Here's how the part is built. I have some questions about the finished solid (model axes, mm). Face numbers are marked on the shaded views. A direction names the side the tool comes from. Give positions to 0.01 mm unless a question says otherwise; leave off trailing zeros. Loops run counter-clockwise (first coordinate to the right, second up) from the corner with the lowest first, then second, coordinate; pieces in that order, holes last. Notation, with made-up numbers: M 43.5,71.5 L 72.5,71.5 A14 ccw 72.5,83.5 Z; hole C 30,-12 d3. An arc over 180 degrees is marked long. Write item = value, one per line. Start each with the question number.
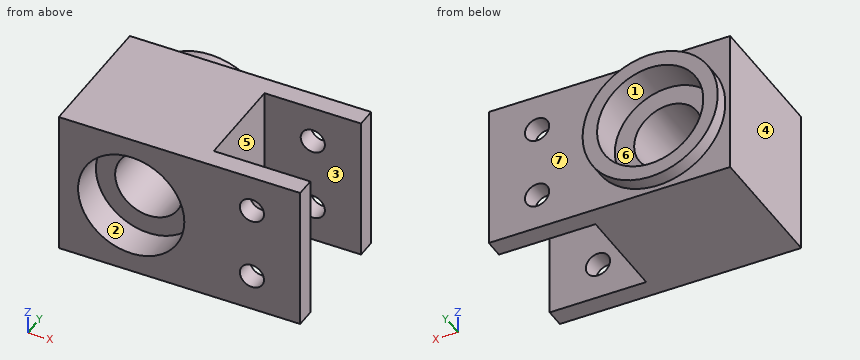
```python
from build123d import *

# Parameters (mm, degrees)
BOSS_EXTRUDE1_DEPTH = 30
SKETCH2_R           = 7
CUT_EXTRUDE1_DEPTH  = 29
SKETCH3_R           = 11
CUT_EXTRUDE2_DEPTH  = 4
SKETCH4_R           = 11
CUT_EXTRUDE3_DEPTH  = 7
SKETCH5_R           = 2.5
CUT_EXTRUDE4_DEPTH  = 29
SKETCH6_R           = 14
SKETCH6_R_2         = 11
BOSS_EXTRUDE2_DEPTH = 3


with BuildPart() as part:
    # Sketch1 → Boss-Extrude1 (new body)
    with BuildSketch(Plane.XY):
        Polygon((10, 10), (10, 14), (-40, 14), (-40, -14), (10, -14), (10, -10), (-10, -10), (-10, 10), align=None)
    extrude(amount=BOSS_EXTRUDE1_DEPTH)

    # Sketch2 → Cut-Extrude1 (cut, through all)
    with BuildSketch(Plane(origin=(0, 14, 0), x_dir=(1, 0, 0), z_dir=(0, 1, 0))):
        with Locations((-25, -15)):
            Circle(SKETCH2_R)
    extrude(amount=-CUT_EXTRUDE1_DEPTH, mode=Mode.SUBTRACT)

    # Sketch3 → Cut-Extrude2 (cut)
    with BuildSketch(Plane(origin=(0, 14, 0), x_dir=(1, 0, 0), z_dir=(0, 1, 0))):
        with Locations((-25, -15)):
            Circle(SKETCH3_R)
    extrude(amount=-CUT_EXTRUDE2_DEPTH, mode=Mode.SUBTRACT)

    # Sketch4 → Cut-Extrude3 (cut)
    with BuildSketch(Plane.XZ.offset(14)):
        with Locations((-25, 15)):
            Circle(SKETCH4_R)
    extrude(amount=-CUT_EXTRUDE3_DEPTH, mode=Mode.SUBTRACT)

    # Sketch5 → Cut-Extrude4 (cut, through all)
    with BuildSketch(Plane(origin=(0, 14, 0), x_dir=(1, 0, 0), z_dir=(0, 1, 0))):
        with Locations((0, -22.5)):
            Circle(SKETCH5_R)
        with Locations((0, -7.5)):
            Circle(SKETCH5_R)
    extrude(amount=-CUT_EXTRUDE4_DEPTH, mode=Mode.SUBTRACT)

    # Sketch6 → Boss-Extrude2 (add)
    with BuildSketch(Plane(origin=(0, 14, 0), x_dir=(1, 0, 0), z_dir=(0, 1, 0))):
        with Locations((-25, -15)):
            Circle(SKETCH6_R)
        with Locations((-25, -15)):
            Circle(SKETCH6_R_2, mode=Mode.SUBTRACT)
    extrude(amount=BOSS_EXTRUDE2_DEPTH)


solid = part.part
```
Q1. If I drill on line 1 along Y through (x, z) = (-1, 18.5); line 2 along Z through (x, y) = (0, 12); line 3 along X through (y, z) = (-11.2, 7.5), over which ranges is the centre line in solid material (lowest first)?
Q2. On a 3-axis mill with a long thin cutter (end or side, diameter ignored), from which of +Z, -Z, +X, -X, +Y, -Y can I reach the whole of each face in a straight line? I mean the marked faces 1, 2 and 3. Say none if no direction works.
Q3. If we section it at D-D, the plane y = 13: List the corners of the cut face in (x, z) for me.
Q4. If we section it at C-C, the plane y = -1.5: List the corners of the cut face in (x, z) for me.
Q5. If we section it at B-B, the plane z = 15: List the corners of the cut face in (x, y) for me, then the cut area to 3 significant figures.
Q6. We'd pull the mould along X, two halves only. Please class the marked faces 4, 5, 6 and 7: pulls with the +X half, pulls with the -X half, needs draft (parallel to the pull), parting line crosses it, or undercut.
Q7. If we section it at A-A, the plane x = -25: List the corners of the cut face in (y, z) for me.
Q8. Will these pins go through, and if not, where does the flat tip stop? pin 1 (1 mm diameter, centred on x = -24, z = 9, fed in from +Y); pin 2 (1 mm diameter, centred on x = -7.5, z = 20, fed in from +Y); pin 3 (6.5 mm diameter, centred on x = -29.5, z = 20, fed in from +Y); pin 4 (6.5 mm diameter, centred on x = -26, z = 10, fed in from -Y).
Resolved:
q1.line_1 = -14 to -10, 10 to 14
q1.line_2 = 0 to 5, 10 to 20, 25 to 30
q1.line_3 = -40 to -33.05, -16.95 to -2.5, 2.5 to 10
q2.face_1 = +Y
q2.face_2 = -Y
q2.face_3 = +Z, -Z, +X
q3.outline = M -40,0 L 10,0 L 10,30 L -40,30 Z; hole C -25,15 d22; hole C 0,7.5 d5; hole C 0,22.5 d5
q4.outline = M -40,0 L -10,0 L -10,30 L -40,30 Z; hole C -25,15 d14
q5.outline = M -40,-14 L -36,-14 L -36,-7 L -32,-7 L -32,10 L -36,10 L -36,17 L -39,17 L -39,14 L -40,14 Z; M -18,-7 L -14,-7 L -14,-14 L 10,-14 L 10,-10 L -10,-10 L -10,10 L 10,10 L 10,14 L -11,14 L -11,17 L -14,17 L -14,10 L -18,10 Z
q5.area = 538 mm²
q6.face_4 = pulls with the -X half
q6.face_5 = pulls with the +X half
q6.face_6 = undercut
q6.face_7 = needs draft
q7.outline = M -14,0 L 14,0 L 14,1 L 17,1 L 17,4 L 10,4 L 10,8 L -7,8 L -7,4 L -14,4 Z; M -14,26 L -7,26 L -7,22 L 10,22 L 10,26 L 17,26 L 17,29 L 14,29 L 14,30 L -14,30 Z
q8.pin_1 = through
q8.pin_2 = 14
q8.pin_3 = 10
q8.pin_4 = -7
